Design review of the part built by this model. Coordinates are the model's own, in mm. Coordinates: 2 decimals unless noted, no trailing zeros. Write each loop counter-clockwise with the first axis right and the second up, starting at its lowest first coordinate (ties: lowest second). Pieces come first, ordered by that corner, then holes.
Q1. Add section A-A, the plane x = -178. Give the boundary of the cut face in (y, z).
Q2. Clearance check with flat-ended pins moving along their axes: pin 1 Ø1.5 at (y, z) = (1457.5, 172) entering from +X; pin 2 Ø13.5 at (x, y) = (-155, 32) entering from +Z; pin 3 Ø22.5 at (x, z) = (-124, 18) entering from +Y; pin 4 Ø16 at (y, z) = (1420, 80) entering from -X. State where each tip first meets the part, or that it passes through.
Q3. Add section B-B, the plane y = 1234.5. Give the boundary of the cut face in (x, z), plus the area to 3 significant figures.
Q4. To check wall thickness, follow probe 1 along Z at (x, y) = (-280, 1420); probe 2 along X at (y, z) = (179.5, 162); probe 3 along Y at (x, z) = (-194.5, 39). State the ranges of each line that lie inside material, in increasing order.
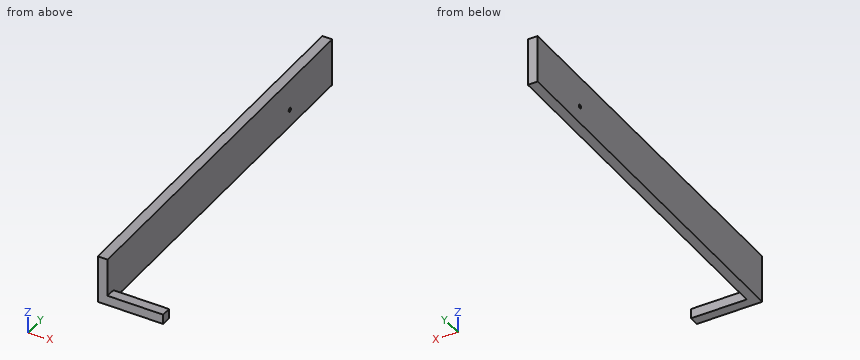
from build123d import *

# Parameters (mm, degrees)
F1_DEPTH = 1750
F0_W     = 255
F0_H     = 45
F2_DEPTH = 45
F3_R     = 9
F4_DEPTH = 300.001


with BuildPart() as f1:
    # F0 (on Front) → F1 (new body)
    with BuildSketch(Plane.XZ):
        Polygon((-300, 0), (-255, 0), (-255, 45), (-255, 220), (-300, 220), align=None)
    extrude(amount=-F1_DEPTH)

    # F0 (on Front) → F2 (join)
    with BuildSketch(Plane.XZ):
        with Locations((-127.5, 22.5)):
            Rectangle(F0_W, F0_H)
    extrude(amount=-F2_DEPTH)

    # F3 (on Right) → F4 (cut, through all)
    with BuildSketch(Plane.YZ):
        with Locations((1420, 80)):
            Circle(F3_R)
    extrude(amount=-F4_DEPTH, mode=Mode.SUBTRACT)


solid = f1.part
Here are the results:
1. outline: (0, 0) - (45, 0) - (45, 45) - (0, 45) - close
2. pin 1: stops at x = -255
2. pin 2: stops at z = 45
2. pin 3: stops at y = 45
2. pin 4: passes through
3. outline: (-300, 0) - (-255, 0) - (-255, 220) - (-300, 220) - close
3. area: 9,900 mm2
4. probe 1: z = 0 to 71, 89 to 220
4. probe 2: x = -300 to -255
4. probe 3: y = 0 to 45
